For this review, take the finished solid that the model builds, in its own axes (mm). A direction names the side the tool comes from. Coordinates: 2 decimals unless noted, no trailing zeros. Loops run counter-clockwise (first coordinate to the right, second up) from the corner with the lowest first, then second, coordinate; pieces in that order, holes last.
1. Take a section at C-C, the plane x = -20.5. State the section outline as (y, z) points, then the cut area to 3 significant figures.
2. Machinability: for faces 1 (the face through (-15, 17, 4)), 2 (the face through (-25, 26, 2)), 3 (the face through (-15, 4, -5)), which of the approach directions +Z, -Z, +X, -X, +Y, -Y give a long, thin tool a straight path to every point of the face, cutting with its end or side? Answer none if there is none.
3. Take a section at A-A, the plane z = -5. State the section outline as (x, y) points.
4. Take a section at B-B, the plane y = 28. State the section outline as (x, z) points, then the cut area to 3 significant figures.
5. Clearance check with flat-ended pins moving along their axes: P1, Ø1, axis at x = -15.5, z = -1, coming from the +Y side; P2, Ø8, axis at x = -10.5, y = 19, coming from the -Z side; P3, Ø8, axis at y = 16.5, z = 2.5, coming from the +X side. State where each tip first meets the part, or that it passes through.
6. Mouldability with a two-part tool opening along Y and no side actions: class faces 4 (the face through (-30, 13, 0.2)), 5 (the face through (-15, 34, 2)), 6 (the face through (-15, 29, 2)) as pulls with the +Y half, pulls with the -Y half, needs draft (parallel to the pull), parting line crosses it, or undercut.
7. To check wall thickness, follow probe 1 along Z at (x, y) = (-7.5, 2.1); probe 2 along Y at (x, z) = (-8.25, -1.5). State the ranges of each line that lie inside material, in increasing order.
8. Take a section at D-D, the plane z = 0.75. State the section outline as (x, y) points, then the cut area to 3 significant figures.
Autodesk Inventor part; units mm, degrees
ref_plane "YZ Plane" through (0, 0, 0) normal (1, 0, 0) x (0, 1, 0)
ref_plane "XZ Plane" through (0, 0, 0) normal (0, 1, 0) x (-1, 0, 0)
ref_plane "XY Plane" through (0, 0, 0) normal (0, 0, 1) x (1, 0, 0)
sketch "Sketch1" plane through (0, 0, 0) normal (0, 1, 0) x (-1, 0, 0)
  line L0 (0, 0) -> (30, 0)
  line L1 (30, 0) -> (30, -10)
  line L2 (30, -10) -> (0, -10)
  line L3 (0, -10) -> (0, 0)
  circle A0 centre (22.5, -5) radius 1.5
  circle A1 centre (7.5, -5) radius 1.5
  dimension "d0" = 3
  dimension "d1" = 3
  dimension "d2" = 30
  dimension "d3" = 15
  dimension "d4" = 5
  dimension "d5" = 10
  dimension "d6" = 7.5
extrude "Extrusion1" add sketch "Sketch1" along normal blind 4
sketch "Sketch2" plane through (0, 4, 0) normal (0, 1, 0) x (1, 0, 0)
  line L0 (-30, 0) -> (0, 0)
  line L1 (0, 0) -> (-30, 0)
  line L2 (-30, 0) -> (-30, -4)
  line L3 (-30, -4) -> (0, -4)
  line L4 (0, -4) -> (0, 0)
  point P0 (-30, 0)
  dimension "d9" = 4
extrude "Extrusion2" add sketch "Sketch2" along normal blind 30 and the other way blind 4
sketch "Sketch3" plane through (-30, 34, 4) normal (0, 0, 1) x (1, 0, 0)
  line L0 (5, -5) -> (25, -5)
  line L1 (25, -5) -> (25, -10)
  line L2 (25, -10) -> (5, -10)
  line L3 (5, -10) -> (5, -5)
  line L4 (0, -34) -> (0, 0)
  line L5 (0, 0) -> (30, 0)
  point P0 (30, -34)
  dimension "d14" = 20
  dimension "d15" = 5
  dimension "d16" = 5
  dimension "d19" = 5
extrude "Extrusion3" cut sketch "Sketch3" against normal blind 30
properties part number "BatteryMount"
Results list:
1. outline: (0, -10) - (4, -10) - (4, 0) - (24, 0) - (24, 4) - (0, 4) - close; (29, 0) - (34, 0) - (34, 4) - (29, 4) - close
1. area: 156 mm2
2. face 1: +Z, +X, -X, +Y, -Y
2. face 2: +Z, -Z
2. face 3: -Z, +X, -X, +Y
3. outline: (-30, 0) - (-24, 0) - (-24, 4) - (-30, 4) - close; (-21, 0) - (-9, 0) - (-9, 4) - (-21, 4) - close; (-6, 0) - (0, 0) - (0, 4) - (-6, 4) - close
4. outline: (-30, 0) - (-25, 0) - (-25, 4) - (-30, 4) - close; (-5, 0) - (0, 0) - (0, 4) - (-5, 4) - close
4. area: 40.0 mm2
5. P1: stops at y = 4
5. P2: stops at z = 0
5. P3: stops at x = 0
6. face 4: needs draft
6. face 5: pulls with the +Y half
6. face 6: undercut
7. probe 1: z = -10 to -6.5, -3.5 to 4
7. probe 2: y = 0 to 4
8. outline: (-30, 0) - (0, 0) - (0, 34) - (-30, 34) - close; hole (-25, 24) - (-5, 24) - (-5, 29) - (-25, 29) - close
8. area: 920 mm2
